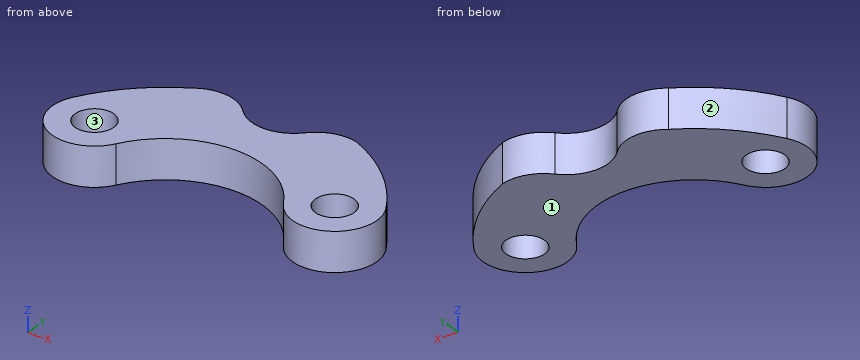
from build123d import *

# Parameters (mm, degrees)
ESQUISSE1_R        = 1.5
BOSS_EXTRU_2_DEPTH = 3


with BuildPart() as part:
    # Esquisse1 → Boss.-Extru.2 (new body)
    with BuildSketch(Plane.XY):
        with BuildLine():
            ThreePointArc((-2.411034891, 11.820685714), (0, 10.75), (2.411034891, 11.820685714))
            ThreePointArc((2.411034891, 11.820685714), (3.975330286, 12.779130538), (5.80943088, 12.737759334))
            ThreePointArc((5.80943088, 12.737759334), (9.414650572, 10.36167721), (12.124355653, 7))
            ThreePointArc((12.124355653, 7), (10.934773091, 2.560417438), (6.495190528, 3.75))
            ThreePointArc((6.495190528, 3.75), (0, 7.5), (-6.495190528, 3.75))
            ThreePointArc((-6.495190528, 3.75), (-10.934773091, 2.560417438), (-12.124355653, 7))
            ThreePointArc((-12.124355653, 7), (-9.780131311, 10.017436376), (-6.707371512, 12.288660114))
            ThreePointArc((-6.707371512, 12.288660114), (-4.47014813, 12.872261577), (-2.411034891, 11.820685714))
        make_face()
        with Locations((9.309773091, 5.375)):
            Circle(ESQUISSE1_R, mode=Mode.SUBTRACT)
        with Locations((-9.309773091, 5.375)):
            Circle(ESQUISSE1_R, mode=Mode.SUBTRACT)
    extrude(amount=BOSS_EXTRU_2_DEPTH)


solid = part.part
Input: part model. Units: mm. Frame: model coordinates. Face numbers are marked on the shaded views. Coordinates: 2 decimals unless noted, no trailing zeros. Loops run counter-clockwise (first coordinate to the right, second up) from the corner with the lowest first, then second, coordinate; pieces in that order, holes last.
Q1. Contact query for flat-ended pins moving along their axis: pin 1 (1 mm diameter, centred on x = -7.5, z = 0.5, fed in from -Y); pin 2 (1.8 mm diameter, centred on x = -9.31, y = 5.38, fed in from -Z); pin 3 (1 mm diameter, centred on y = 6, z = 2.5, fed in from +X). Output: stop coordinate, or through.
Q2. Draft query along X for the marked faces 1, 2 and 3. Return one class per face: +X half, -X half, draft (parallel to the pull), parting line (faces both ways), or undercut.
Q3. Material intervals for line 1 (X direction, y = 6.75, z = 1.15); line 2 (Y direction, x = 10.25, z = 2.2); line 3 (X direction, y = 3.75, z = 2.8), sorted ascending.
Q4. Cut plane C-C (z = 0.4). Output: boundary loops of the cut face in (x, y) (3 decimals).
Q5. Cut plane D-D (x = 9.5). Output: boundary loops of the cut face in (y, z).
Q6. Cut plane B-B (y = 6.5). Output: boundary loops of the cut face in (x, z), then the cut area to 3 significant figures.
Q7. Cut plane A-A (x = -8.75). Output: boundary loops of the cut face in (y, z), then the cut area to 3 significant figures.
Working result:
1. pin 1: stops at y = 2.4
1. pin 2: passes through
1. pin 3: stops at x = 12.56
2. face 1: draft
2. face 2: -X half
2. face 3: undercut
3. line 1: x = -12.25 to -9.91, -8.71 to -3.27, 3.27 to 8.71, 9.91 to 12.25
3. line 2: y = 2.26 to 4.21, 6.54 to 9.54
3. line 3: x = -12.12 to -6.5, 6.5 to 12.12
4. outline: (-12.124, 7) arc R3.25 ccw to (-6.495, 3.75) arc R7.5 cw to (6.495, 3.75) arc R3.25 ccw to (12.124, 7) arc R14 ccw to (5.809, 12.738) arc R3.25 ccw to (2.411, 11.821) arc R3.25 cw to (-2.411, 11.821) arc R3.25 ccw to (-6.707, 12.289) arc R14 ccw to start; hole circle Ø3 at (-9.31, 5.375); hole circle Ø3 at (9.31, 5.375)
5. outline: (2.13, 0) - (3.89, 0) - (3.89, 3) - (2.13, 3) - close; (6.86, 0) - (10.28, 0) - (10.28, 3) - (6.86, 3) - close
6. outline: (-12.36, 0) - (-10.3, 0) - (-10.3, 3) - (-12.36, 3) - close; (-8.32, 0) - (-3.74, 0) - (-3.74, 3) - (-8.32, 3) - close; (3.74, 0) - (8.32, 0) - (8.32, 3) - (3.74, 3) - close; (10.3, 0) - (12.36, 0) - (12.36, 3) - (10.3, 3) - close
6. area: 39.8 mm2
7. outline: (2.17, 0) - (3.98, 0) - (3.98, 3) - (2.17, 3) - close; (6.77, 0) - (10.93, 0) - (10.93, 3) - (6.77, 3) - close
7. area: 17.9 mm2
